```python
from build123d import *

# Parameters (mm, degrees)
SZKIC1_R                    = 4
SZKIC1_R_2                  = 1.5
DODANIE_WYCI_GNI_CIE1_DEPTH = 5
SZKIC1_3_R                  = 36
DODANIE_WYCI_GNI_CIE2_DEPTH = 25
ZAOKR_GLENIE1_R             = 10
ZAOKR_GLENIE2_R             = 2
SZKIC3_R                    = 3
WYTNIJ_WYCI_GNI_CIE2_DEPTH  = 52.5
WYTNIJ_WYCI_GNI_CIE3_DEPTH  = 6
WYTNIJ_WYCI_GNI_CIE4_DEPTH  = 26
WYTNIJ_WYCI_GNI_CIE5_DEPTH  = 26
DODANIE_WYCI_GNI_CIE3_DEPTH = 25


with BuildPart() as part:
    # Szkic1 → Dodanie-wyci_gni_cie1 (new body)
    with BuildSketch(Plane(origin=(0, 0, 0), x_dir=(1, 0, 0), z_dir=(0, 1, 0))):
        Polygon((-20.5, -48.6036745), (-39.5, 60.773175281), (-39.5, 136.3963255), (-13, 156.3963255), (-13, 211.3963255), (12, 211.3963255), (12, 156.3963255), (38.5, 136.3963255), (38.5, 60.773175281), (19.5, -48.6036745), align=None)
        with Locations((-0.5, 105.3963255)):
            Circle(SZKIC1_R, mode=Mode.SUBTRACT)
        with Locations((-0.5, 97.3963255)):
            Circle(SZKIC1_R_2, mode=Mode.SUBTRACT)
        with Locations((-8.5, 105.3963255)):
            Circle(SZKIC1_R_2, mode=Mode.SUBTRACT)
        with Locations((-0.5, 113.3963255)):
            Circle(SZKIC1_R_2, mode=Mode.SUBTRACT)
        with Locations((7.5, 105.3963255)):
            Circle(SZKIC1_R_2, mode=Mode.SUBTRACT)
        with BuildLine():
            Line((-25.198683142, 138.122080663), (-26.54670895, 139.908214858))
            Line((-26.54670895, 139.908214858), (-11.466042799, 151.289849688))
            Line((-11.466042799, 151.289849688), (10.466042799, 151.289849688))
            Line((10.466042799, 151.289849688), (25.54670895, 139.908214858))
            Line((25.54670895, 139.908214858), (24.198683142, 138.122080663))
            ThreePointArc((24.198683142, 138.122080663), (-0.5, 146.3963255), (-25.198683142, 138.122080663))
        make_face(mode=Mode.SUBTRACT)
    extrude(amount=DODANIE_WYCI_GNI_CIE1_DEPTH)

    # Szkic1_3 → Dodanie-wyci_gni_cie2 (add)
    with BuildSketch(Plane(origin=(0, 0, 0), x_dir=(1, 0, 0), z_dir=(0, 1, 0))):
        Polygon((-39.5, 60.773175281), (-20.5, -48.6036745), (19.5, -48.6036745), (38.5, 60.773175281), (38.5, 136.3963255), (12, 156.3963255), (12, 211.3963255), (-13, 211.3963255), (-13, 156.3963255), (-39.5, 136.3963255), align=None)
        with Locations((-0.5, 105.3963255)):
            Circle(SZKIC1_3_R, mode=Mode.SUBTRACT)
        with BuildLine():
            ThreePointArc((24.198683142, 138.122080663), (-0.5, 146.3963255), (-25.198683142, 138.122080663))
            Line((-25.198683142, 138.122080663), (-26.54670895, 139.908214858))
            Line((-26.54670895, 139.908214858), (-11.466042799, 151.289849688))
            Line((-11.466042799, 151.289849688), (10.466042799, 151.289849688))
            Line((10.466042799, 151.289849688), (25.54670895, 139.908214858))
            Line((25.54670895, 139.908214858), (24.198683142, 138.122080663))
        make_face(mode=Mode.SUBTRACT)
    extrude(amount=DODANIE_WYCI_GNI_CIE2_DEPTH)

    # Zaokr_glenie1
    zaokr_glenie1_edges = [part.edges().sort_by_distance(p)[0] for p in [
        (-0.5, 25, -211.3963255),
    ]]
    fillet(zaokr_glenie1_edges, radius=ZAOKR_GLENIE1_R)

    # Zaokr_glenie2
    zaokr_glenie2_edges = [part.edges().sort_by_distance(p)[0] for p in [
        (-0.5, 0, -211.3963255),
    ]]
    fillet(zaokr_glenie2_edges, radius=ZAOKR_GLENIE2_R)

    # Szkic3 → Wytnij-wyci_gni_cie2 (cut, through all)
    with BuildSketch(Plane.ZY.offset(13)):
        with Locations((-199.3963255, 12)):
            Circle(SZKIC3_R)
    extrude(amount=-WYTNIJ_WYCI_GNI_CIE2_DEPTH, mode=Mode.SUBTRACT)

    # Szkic4 → Wytnij-wyci_gni_cie3 (cut, through all)
    with BuildSketch(Plane(origin=(0, 5, 0), x_dir=(1, 0, 0), z_dir=(0, 1, 0))):
        with BuildLine():
            ThreePointArc((-7.5, 117.520681153), (-5.449747468, 118.492126353), (-3.269507466, 119.119657034))
            Line((-3.269507466, 119.119657034), (-25.071343028, 131.706952664))
            ThreePointArc((-25.071343028, 131.706952664), (-34.345756663, 117.66273312), (-36.222813233, 100.937557201))
            Line((-36.222813233, 100.937557201), (-7.5, 117.520681153))
        make_face()
        with BuildLine():
            ThreePointArc((6.5, 117.520681153), (8.366422488, 116.230832976), (10, 114.656455088))
            Line((10, 114.656455088), (10, 139.831046349))
            ThreePointArc((10, 139.831046349), (-6.799857719, 140.84081439), (-22.222813233, 134.103805104))
            Line((-22.222813233, 134.103805104), (6.5, 117.520681153))
        make_face()
        with BuildLine():
            Line((13.5, 138.562573403), (13.5, 105.3963255))
            ThreePointArc((13.5, 105.3963255), (13.316169956, 103.135032123), (12.769507466, 100.933123554))
            Line((12.769507466, 100.933123554), (34.571343028, 113.520419185))
            ThreePointArc((34.571343028, 113.520419185), (27.045898944, 128.57440677), (13.5, 138.562573403))
        make_face()
        with BuildLine():
            Line((35.222813233, 109.855093798), (6.5, 93.271969847))
            ThreePointArc((6.5, 93.271969847), (4.449747468, 92.300524646), (2.269507466, 91.672993965))
            Line((2.269507466, 91.672993965), (24.071343028, 79.085698335))
            ThreePointArc((24.071343028, 79.085698335), (32.519451457, 91.05352851), (35.5, 105.3963255))
            ThreePointArc((35.5, 105.3963255), (35.430636485, 107.630013439), (35.222813233, 109.855093798))
        make_face()
        with BuildLine():
            Line((21.222813233, 76.688845895), (-7.5, 93.271969847))
            ThreePointArc((-7.5, 93.271969847), (-9.366422488, 94.561818023), (-11, 96.136195911))
            Line((-11, 96.136195911), (-11, 70.96160465))
            ThreePointArc((-11, 70.96160465), (5.799857719, 69.951836609), (21.222813233, 76.688845895))
        make_face()
        with BuildLine():
            ThreePointArc((-14.5, 105.3963255), (-14.316169956, 107.657618877), (-13.769507466, 109.859527445))
            Line((-13.769507466, 109.859527445), (-35.571343028, 97.272231814))
            ThreePointArc((-35.571343028, 97.272231814), (-28.045898944, 82.218244229), (-14.5, 72.230077596))
            Line((-14.5, 72.230077596), (-14.5, 105.3963255))
        make_face()
    extrude(amount=-WYTNIJ_WYCI_GNI_CIE3_DEPTH, mode=Mode.SUBTRACT)

    # Szkic5 → Wytnij-wyci_gni_cie4 (cut, through all)
    with BuildSketch(Plane(origin=(0, 25, 0), x_dir=(1, 0, 0), z_dir=(0, 1, 0))):
        Polygon((-0.5, 167.537901521), (-3.188590085, 162.617610716), (2.188590085, 162.617610716), align=None)
        Polygon((-8, 162.617610716), (-6.037476669, 162.617610716), (-1.924443292, 170.144723317), (-8, 181.2633784), align=None)
        Polygon((0.924443292, 170.144723317), (5.037476669, 162.617610716), (7, 162.617610716), (7, 181.2633784), align=None)
        Polygon((-8, 186.477021992), (-0.5, 172.751545113), (7, 186.477021992), (7, 190.068564472), (-8, 190.068564472), align=None)
    extrude(amount=-WYTNIJ_WYCI_GNI_CIE4_DEPTH, mode=Mode.SUBTRACT)

    # Szkic6 → Wytnij-wyci_gni_cie5 (cut, through all)
    with BuildSketch(Plane(origin=(0, 25, 0), x_dir=(1, 0, 0), z_dir=(0, 1, 0))):
        Polygon((-3.890112786, 35.914234697), (-36.243006097, 71.238147911), (-25.927207854, 11.853436604), align=None)
        Polygon((2.890112786, 35.914234697), (24.927207854, 11.853436604), (35.243006097, 71.238147911), align=None)
        Polygon((2.931825406, -17.721341562), (17.161306881, -32.852341508), (23.609193637, 4.266055389), align=None)
        Polygon((-0.5, -21.370592599), (-17.091150305, -39.01288651), (-16.206822662, -44.1036745), (15.206822662, -44.1036745), (16.091150305, -39.01288651), align=None)
        Polygon((-3.931825406, -17.721341562), (-24.609193637, 4.266055389), (-18.161306881, -32.852341508), align=None)
        Polygon((20.976041499, 8.764580183), (-0.5, 32.212802226), (-21.976041499, 8.764580183), (-0.5, -14.072090524), align=None)
        with BuildLine():
            Line((-0.5, 39.615667168), (30.262410293, 73.203040667))
            ThreePointArc((30.262410293, 73.203040667), (-0.5, 60.868430026), (-31.262410293, 73.203040667))
            Line((-31.262410293, 73.203040667), (-0.5, 39.615667168))
        make_face()
    extrude(amount=-WYTNIJ_WYCI_GNI_CIE5_DEPTH, mode=Mode.SUBTRACT)

    # Szkic7 → Dodanie-wyci_gni_cie3 (add)
    with BuildSketch(Plane.XZ):
        with BuildLine():
            Line((40.5, -128.178388263), (40.5, -85.340764579))
            add(Edge.make_bspline(
                [(40.5, -85.340764579), (40.5, -72.286527889), (38.5, -60.773175281)],
                knots=[1.478281608, 1.478281608, 1.478281608, 2.061293097, 2.061293097, 2.061293097], degree=2, weights=[1, 0.957812218, 1]))
            Line((38.5, -60.773175281), (38.5, -136.3963255))
            add(Edge.make_bspline(
                [(38.5, -136.3963255), (40.5, -134.886891537), (40.5, -128.178388263)],
                knots=[3.382541088, 3.382541088, 3.382541088, 4.954548483, 4.954548483, 4.954548483], degree=2, weights=[1, 0.706678474, 1]))
        make_face()
        with BuildLine():
            Line((-39.5, -136.3963255), (-39.5, -60.773175281))
            add(Edge.make_bspline(
                [(-39.5, -60.773175281), (-41.5, -72.286527889), (-41.5, -85.340764579)],
                knots=[4.22189221, 4.22189221, 4.22189221, 4.804903699, 4.804903699, 4.804903699], degree=2, weights=[1, 0.957812218, 1]))
            Line((-41.5, -85.340764579), (-41.5, -128.178388263))
            add(Edge.make_bspline(
                [(-41.5, -128.178388263), (-41.5, -134.886891537), (-39.5, -136.3963255)],
                knots=[1.328636824, 1.328636824, 1.328636824, 2.900644219, 2.900644219, 2.900644219], degree=2, weights=[1, 0.706678474, 1]))
        make_face()
    extrude(amount=-DODANIE_WYCI_GNI_CIE3_DEPTH)


solid = part.part
```
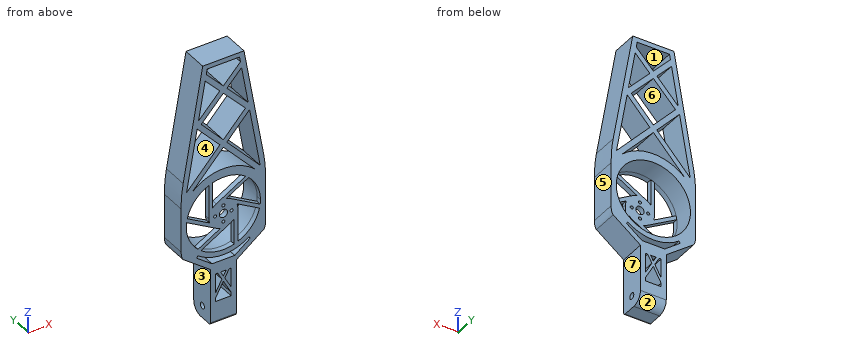
Work out the finished part from the listing and answer in its coordinate system (mm). Face numbers are marked on the shaded views. A direction names the side the tool comes from. Round coordinates to 2 decimals unless told otherwise and drop trailing zeros.
(1) The mould has two halves that part along X. Classify the marked faces 1, 2, 3 and 4: pulls with the +X half, pulls with the -X half, needs draft (parallel to the pull), parting line crosses it, or undercut.
Computed values:
face 1: undercut
face 2: needs draft
face 3: pulls with the -X half
face 4: undercut
(2) Find the intervals of material crossed by L1, parallel to X at y = 4.5, z = 23; L2, parallel to X at y = 11, z = -181.5; L3, parallel to X at y = 23.5, z = -97.5, in increasing order.
Computed values:
L1: x = -24.95 to -19.87, -8.9 to -2.03, 1.03 to 7.9, 18.87 to 23.95
L2: x = -13 to -5.28, 4.28 to 12
L3: x = -41.5 to -35.62, 34.62 to 40.5
(3) Each of these flat-tipped pins is pushed along its axis until it touches: P1, Ø1, axis at y = 16.5, z = -50.5, coming from the +X side; P2, Ø5, axis at y = 16, z = -150, coming from the -X side; P3, Ø12, axis at y = 13.5, z = -43, coming from the -X side; P4, Ø2.5, axis at x = -0.5, z = -113.4, coming from the -Y side. Where does it stop, or does it pass through?
Computed values:
P1: stops at x = 36.8
P2: stops at x = -24.79
P3: stops at x = -37.45
P4: passes through
(4) The part is cut by section A-A, the plane y = 12. Give the number of separate pieces and of enclosed holes in the cut face, and give its area (3 significant figures).
Computed values:
separate pieces: 2
enclosed holes: 13
area: 6,120 mm2
(5) For the marked faces 5, 6 and 7, determine the directions among +Z, -Z, +X, -X, +Y, -Y from which every point of the face is accessible in a straight line to the end or side of a thin tool.
Computed values:
face 5: +Z, -Z, +X, +Y, -Y
face 6: +Y, -Y
face 7: -Z, +X, +Y, -Y
